from build123d import *

# Parameters (mm, degrees)
F0_W     = 50.8
F0_H     = 31.75
F1_DEPTH = 31.75
F2_W     = 19.062214
F2_H     = 19.023106
F3_DEPTH = 19.05
F4_W     = 19.062212
F4_H     = 19.023106
F5_DEPTH = 19.05
F7_DEPTH = 25.4
F9_DEPTH = 25.4


with BuildPart() as f1:
    # F0 (on Front) → F1 (new body)
    with BuildSketch(Plane.XZ):
        with Locations((-33.25202, 44.606277)):
            Rectangle(F0_W, F0_H)
    extrude(amount=F1_DEPTH)

    # F2 (on face) → F3 (cut)
    with BuildSketch(Plane(origin=(-58.65202, 0, 0), x_dir=(0, -1, 0), z_dir=(-1, 0, 0))):
        with Locations((9.531107, 50.969724)):
            Rectangle(F2_W, F2_H)
    extrude(amount=-F3_DEPTH, mode=Mode.SUBTRACT)

    # F4 (on face) → F5 (cut)
    with BuildSketch(Plane.YZ.offset(-7.85202)):
        with Locations((-9.531106, 50.969724)):
            Rectangle(F4_W, F4_H)
    extrude(amount=-F5_DEPTH, mode=Mode.SUBTRACT)

    # F6 (on face) → F7 (cut)
    with BuildSketch(Plane(origin=(0, -19.062214, 0), x_dir=(-1, 0, 0), z_dir=(0, 1, 0))):
        Polygon((41.800097, 60.481277), (58.65202, 41.458171), (58.65202, 60.481277), align=None)
    extrude(amount=-F7_DEPTH, mode=Mode.SUBTRACT)

    # F8 (on face) → F9 (cut)
    with BuildSketch(Plane.YZ.offset(-26.90202)):
        Polygon((-16.839711, 60.481277), (0, 41.458171), (0, 60.481277), align=None)
    extrude(amount=-F9_DEPTH, mode=Mode.SUBTRACT)


solid = f1.part
The model under review builds one solid part; all positions refer to its coordinate system, in mm. A direction names the side the tool comes from. Coordinates: 2 decimals unless noted, no trailing zeros. Order: outer loops, then holes, each group sorted by start corner. A loop starts at its lowest first (then second) coordinate and runs counter-clockwise, first axis right, second up. Notation, with made-up numbers: (9.25, 51.5) -> (51.25, 51.5) arc R27 ccw to (51.25, 68.5) -> close; hole circle Ø9 at (49.5, 31.25). An arc over 180 degrees is marked (long way). Answer in a Markdown table with one row per item.
(1) Consider section B-B (y = -21.5). Write out the cut boundary in (x, z), plus the area to 3 significant figures.
Answers:
| item | result |
|---|---|
| outline | (-58.65, 28.73) -> (-7.85, 28.73) -> (-7.85, 60.48) -> (-41.8, 60.48) -> (-58.65, 41.46) -> close |
| area | 1,450 mm² |
(2) Insertion check: pin 1 (15 mm diameter, centred on x = -14, y = -6, fed in from +Z); pin 2 (5.5 mm diameter, centred on x = -15, z = 51.5, fed in from +Y); pin 3 (8 mm diameter, centred on x = -38.5, y = -5, fed in from +Z). Each pin has a flat end and moves straight along its axis. Give the tip position at first contact, or say it passes through.
Answers:
| item | result |
|---|---|
| pin 1 | z = 41.46 |
| pin 2 | y = -19.06 |
| pin 3 | z = 51.63 |
(3) Consider section A-A (x = -24.5). Write out the cut boundary in (y, z).
Answers:
| item | result |
|---|---|
| outline | (-31.75, 28.73) -> (0, 28.73) -> (0, 41.46) -> (-19.06, 41.46) -> (-19.06, 60.48) -> (-31.75, 60.48) -> close |
(4) Consider section C-C (z = 46). Write out the cut boundary in (x, y), plus the area to 3 significant figures.
Answers:
| item | result |
|---|---|
| outline | (-54.63, -31.75) -> (-7.85, -31.75) -> (-7.85, -19.06) -> (-26.9, -19.06) -> (-26.9, -4.02) -> (-39.6, -4.02) -> (-39.6, -19.06) -> (-54.63, -19.06) -> close |
| area | 785 mm² |
(5) Wall thickness on line 1 along Y through (x, z) = (-18.5, 49.5); line 2 along Z through (x, y) = (-51, -10); line 3 along Z through (x, y) = (-38, -14.5): over which ranges is each line inside the solid? List them lowest first.
Answers:
| item | result |
|---|---|
| line 1 | -31.75 to -19.06 |
| line 2 | 28.73 to 41.46 |
| line 3 | 28.73 to 57.84 |
(6) Machinability: for faces 1 (the flat face through (-58.652, -16, 35)), 2 (the flat face through (-39.602, -12, 49)), 3 (the flat face through (-26.902, -12, 49)), which of the approach directions +Z, -Z, +X, -X, +Y, -Y give a long, thin tool a straight path to every point of the face, cutting with its end or side? Answer none if there is none.
Answers:
| item | result |
|---|---|
| face 1 | +Z, -Z, -X, +Y, -Y |
| face 2 | +Z, -X, +Y |
| face 3 | +Z, +X, +Y |
(7) Consider section D-D (y = -11). Write out the cut boundary in (x, z).
Answers:
| item | result |
|---|---|
| outline | (-58.65, 28.73) -> (-7.85, 28.73) -> (-7.85, 41.46) -> (-26.9, 41.46) -> (-26.9, 53.88) -> (-39.6, 53.88) -> (-39.6, 41.46) -> (-58.65, 41.46) -> close |
